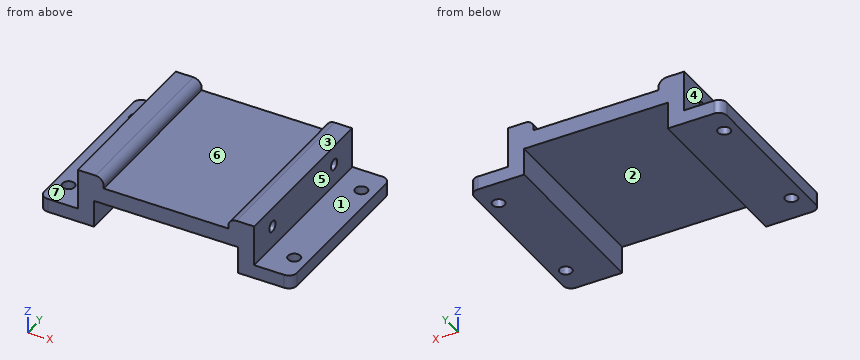
from build123d import *

# Parameters (mm, degrees)
SKETCH1_W             = 20
SKETCH1_H             = 63.5
BOSS_EXTRUDE1_DEPTH   = 5
BOSS_EXTRUDE1_2_DEPTH = 5
SKETCH2_W             = 6
SKETCH2_H             = 63.5
BOSS_EXTRUDE2_DEPTH   = 15
BOSS_EXTRUDE3_REACH   = 74.7
SKETCH3_W             = 6
SKETCH3_H             = 63.5
SKETCH4_W             = 4
SKETCH4_H             = 63.5
BOSS_EXTRUDE4_DEPTH   = 3.5
SKETCH6_R             = 2.25
CUT_EXTRUDE2_DEPTH    = 6
FILLET1_R             = 3
SKETCH7_R             = 2
CUT_EXTRUDE6_DEPTH    = 15


with BuildPart() as part:
    # Sketch1 → Boss-Extrude1 (new body)
    with BuildSketch(Plane.XY):
        with Locations((-36.35, 0)):
            Rectangle(SKETCH1_W, SKETCH1_H)
    extrude(amount=BOSS_EXTRUDE1_DEPTH)



with BuildPart() as body_2:
    # Sketch1 → Boss-Extrude1 2 (new body)
    with BuildSketch(Plane.XY):
        with Locations((36.35, 0)):
            Rectangle(SKETCH1_W, SKETCH1_H)
    extrude(amount=BOSS_EXTRUDE1_2_DEPTH)


with BuildPart() as part_1:
    add(part.part)

    add(body_2.part)  # Boss-Extrude2 merges body 2
    # Sketch2 → Boss-Extrude2 (add)
    with BuildSketch(Plane.XY.offset(5)):
        with Locations((-29.35, 0)):
            Rectangle(SKETCH2_W, SKETCH2_H)
        with Locations((29.35, 0)):
            Rectangle(SKETCH2_W, SKETCH2_H)
    extrude(amount=BOSS_EXTRUDE2_DEPTH)

    # Sketch3 → Boss-Extrude3 (add, up to next)
    with BuildSketch(Plane(origin=(-26.35, 0, 0), x_dir=(0, 0, -1), z_dir=(1, 0, 0)), mode=Mode.PRIVATE) as boss_extrude3_sk1:
        with Locations((-13, 0)):
            Rectangle(SKETCH3_W, SKETCH3_H)
    boss_extrude3_tool1 = extrude(boss_extrude3_sk1.sketch, amount=BOSS_EXTRUDE3_REACH, mode=Mode.PRIVATE) - part_1.part
    add(boss_extrude3_tool1.solids().sort_by_distance((-26.35, 0, 13))[0])

    # Sketch4 → Boss-Extrude4 (add)
    with BuildSketch(Plane(origin=(-26.35, 0, 0), x_dir=(0, 0, -1), z_dir=(1, 0, 0))):
        with Locations((-18, 0)):
            Rectangle(SKETCH4_W, SKETCH4_H)
    boss_extrude4 = extrude(amount=BOSS_EXTRUDE4_DEPTH)

    # Mirror1: Boss-Extrude4 across plane
    add(boss_extrude4.mirror(Plane(origin=(0, 0, 0), x_dir=(0, 0, 1), z_dir=(1, 0, 0))))

    # Sketch6 → Cut-Extrude2 (cut, through all)
    with BuildSketch(Plane.XY.offset(5)):
        with Locations((-41.35, 21.75)):
            Circle(SKETCH6_R)
        with Locations((-41.35, -21.75)):
            Circle(SKETCH6_R)
        with Locations((41.35, -21.75)):
            Circle(SKETCH6_R)
        with Locations((41.35, 21.75)):
            Circle(SKETCH6_R)
    extrude(amount=-CUT_EXTRUDE2_DEPTH, mode=Mode.SUBTRACT)

    # Fillet1
    fillet1_edges = [part_1.edges().sort_by_distance(p)[0] for p in [
        (46.35, 31.75, 2.5),
        (46.35, -31.75, 2.5),
        (-22.85, 0, 20),
        (22.85, 0, 20),
        (-46.35, 31.75, 2.5),
        (-46.35, -31.75, 2.5),
    ]]
    fillet(fillet1_edges, radius=FILLET1_R)

    # Sketch7 → Cut-Extrude6 (cut)
    with BuildSketch(Plane.ZY.offset(32.35)):
        with Locations((13, 20)):
            Circle(SKETCH7_R)
        with Locations((13, -20)):
            Circle(SKETCH7_R)
    cut_extrude6 = extrude(amount=-CUT_EXTRUDE6_DEPTH, mode=Mode.SUBTRACT)

    # Mirror2: Cut-Extrude6 across plane
    add(cut_extrude6.mirror(Plane(origin=(0, 0, 0), x_dir=(0, 0, 1), z_dir=(1, 0, 0))), mode=Mode.SUBTRACT)


solid = part_1.part
Geometry check sheet. Reference: the model listing, model coordinates, mm. Face numbers are marked on the shaded views. A direction names the side the tool comes from. Give positions to 0.01 mm unless a question says otherwise; leave off trailing zeros. Write each loop counter-clockwise with the first axis right and the second up, starting at its lowest first coordinate (ties: lowest second). Pieces come first, ordered by that corner, then holes. Notation, with made-up numbers: M 69,16 L 101,16 A4 cw 101,22 Z; hole C 77,-31 d11. An arc over 180 degrees is marked long. Answer as CSV lines item,"result". Start each with the question number.
Q1. Material ranges on L1, parallel to Y at x = 21.5, z = 13; L2, parallel to Y at x = -41.35, z = 2.3; L3, parallel to X at y = -26.5, z = 17, recorded low to high.
Q2. Tool access check on the marked faces 1, 2, 3 and 4. Record the directions out of +Z, -Z, +X, -X, +Y, -Y that give a thin tool (end or side, any length) a straight path to the whole face; none if there is none.
Q3. Section check B-B, the plane x = -41.35. Record the cut outline in (y, z).
Q4. Release check for a two-part mould opening along X. For the marked faces 5, 6 and 7 record: pulls with the +X half, pulls with the -X half, needs draft (parallel to the pull), parting line crosses it, or undercut.
Q5. Section check C-C, the plane y = -25.5. Record the cut outline in (x, z), then the cut area to 3 significant figures.
Q6. Section check A-A, the plane z = 4. Record the cut outline in (x, y).
Q7. Section check D-D, the plane z = 13. Record the cut outline in (x, y), then the cut area to 3 significant figures.
Q8. Go/stop test with flat-tipped pins: pin 1 (3 mm diameter, centred on x = -15, y = 21.5, fed in from +Z); pin 2 (6.5 mm diameter, centred on y = -20, z = 13, fed in from -X); pin 3 (3.5 mm diameter, centred on y = 20, z = 13, fed in from +X). Record where each tip stops, or that it passes through.
Geometry says:
1,L1,"-31.75 to -22, -18 to 18, 22 to 31.75"
1,L2,"-31.75 to -24, -19.5 to 19.5, 24 to 31.75"
1,L3,"-32.35 to -22.85, 22.85 to 32.35"
2,face 1,"+Z, +X, +Y, -Y"
2,face 2,"-Z, +Y, -Y"
2,face 3,"+Z, +X, -X, +Y, -Y"
2,face 4,"+Z, -X, +Y, -Y"
3,outline,"M -31.75,0 L -24,0 L -24,5 L -31.75,5 Z; M -19.5,0 L 19.5,0 L 19.5,5 L -19.5,5 Z; M 24,0 L 31.75,0 L 31.75,5 L 24,5 Z"
4,face 5,"pulls with the +X half"
4,face 6,"undercut"
4,face 7,"needs draft"
5,outline,"M -46.35,0 L -26.35,0 L -26.35,10 L 26.35,10 L 26.35,0 L 46.35,0 L 46.35,5 L 32.35,5 L 32.35,20 L 25.85,20 A3 ccw 22.85,17 L 22.85,16 L -22.85,16 L -22.85,17 A3 ccw -25.85,20 L -32.35,20 L -32.35,5 L -46.35,5 Z"
5,area,"720 mm^2"
6,outline,"M -46.35,-28.75 A3 ccw -43.35,-31.75 L -26.35,-31.75 L -26.35,31.75 L -43.35,31.75 A3 ccw -46.35,28.75 Z; M 26.35,-31.75 L 43.35,-31.75 A3 ccw 46.35,-28.75 L 46.35,28.75 A3 ccw 43.35,31.75 L 26.35,31.75 Z; hole C -41.35,-21.75 d4.5; hole C -41.35,21.75 d4.5; hole C 41.35,-21.75 d4.5; hole C 41.35,21.75 d4.5"
7,outline,"M -32.35,-31.75 L 32.35,-31.75 L 32.35,-22 L 17.35,-22 L 17.35,-18 L 32.35,-18 L 32.35,18 L 17.35,18 L 17.35,22 L 32.35,22 L 32.35,31.75 L -32.35,31.75 L -32.35,22 L -17.35,22 L -17.35,18 L -32.35,18 L -32.35,-18 L -17.35,-18 L -17.35,-22 L -32.35,-22 Z"
7,area,"3,870 mm^2"
8,pin 1,"z = 16"
8,pin 2,"x = -32.35"
8,pin 3,"x = 17.35"
